Input: part model. Units: mm. Frame: model coordinates. Give positions to 0.01 mm unless a question says otherwise; leave off trailing zeros. Order: outer loops, then holes, each group sorted by start corner. A loop starts at its lowest first (then second) coordinate and runs counter-clockwise, first axis right, second up.
```python
from build123d import *

# Parameters (mm, degrees)
SKETCH1_R           = 1
BOSS_EXTRUDE1_DEPTH = 4.1


with BuildPart() as part:
    # Sketch1 → Boss-Extrude1 (new body)
    with BuildSketch(Plane(origin=(0, 0, 0), x_dir=(1, 0, 0), z_dir=(0, 1, 0))):
        with BuildLine():
            Line((-47.45, -31.685353535), (-47.45, -76.685353535))
            Line((-47.45, -76.685353535), (47.45, -76.685353535))
            Line((47.45, -76.685353535), (47.45, -31.685353535))
            ThreePointArc((47.45, -31.685353535), (0, -14.620077353), (-47.45, -31.685353535))
        make_face()
        with Locations((0, -71.260285785)):
            Circle(SKETCH1_R, mode=Mode.SUBTRACT)
    extrude(amount=BOSS_EXTRUDE1_DEPTH)


solid = part.part
```
1) Cut plane B-B (y = 2). Return the cut outline in (x, z), then the cut area to 3 significant figures.
2) Cut plane D-D (x = 32). Return the cut outline in (y, z).
3) Line query: probe 1 along Z at (x, y) = (0, 2.6); probe 2 along X at (y, z) = (3.75, 72); probe 3 along Z at (x, y) = (-44, 0.3). Output: solid intervals per line, ascending.
4) Pull-direction query (X, two-part tool) for faces 1 (the face through (47.45, 2, 55)), 2 (the face through (-47.45, 2, 54)), 3 (the face through (-1, 0, 45)), 4 (the face through (-0.13, 2.02, 70.27)); classes: pulls with the +X half, pulls with the -X half, needs draft (parallel to the pull), parting line crosses it, or undercut.
5) First-contact query: P1, Ø1, axis at x = -38, y = 2.5, coming from the -Z side; P2, Ø1.5, axis at y = 1, z = 26.5, coming from the -X side. Flat tips, straight axial feed; report the tip coordinate or a pass-through.
6) Cut plane C-C (z = 24). Return the cut outline in (x, y), then the cut area to 3 significant figures.
7) Cut plane A-A (x = 0). Return the cut outline in (y, z).
Geometry says:
1. outline: (-47.45, 31.69) arc R74.5 ccw to (47.45, 31.69) - (47.45, 76.69) - (-47.45, 76.69) - close; hole circle Ø2 at (0, 71.26)
1. area: 5,370 mm2
2. outline: (0, 21.84) - (4.1, 21.84) - (4.1, 76.69) - (0, 76.69) - close
3. probe 1: z = 14.62 to 70.26, 72.26 to 76.69
3. probe 2: x = -47.45 to -0.67, 0.67 to 47.45
3. probe 3: z = 29 to 76.69
4. face 1: pulls with the +X half
4. face 2: pulls with the -X half
4. face 3: needs draft
4. face 4: undercut
5. P1: stops at z = 24.75
5. P2: stops at x = -41.5
6. outline: (-36.19, 0) - (36.19, 0) - (36.19, 4.1) - (-36.19, 4.1) - close
6. area: 297 mm2
7. outline: (0, 14.62) - (4.1, 14.62) - (4.1, 70.26) - (0, 70.26) - close; (0, 72.26) - (4.1, 72.26) - (4.1, 76.69) - (0, 76.69) - close
